```python
from build123d import *

# Parameters (mm, degrees)
F0_W      = 48.26
F0_H      = 35.56
F0_R      = 1.5
F1_DEPTH  = 2
F2_W      = 48.329203
F2_H      = 2
F3_DEPTH  = 25
F5_W      = 18
F5_H      = 9
F6_DEPTH  = 25
F7_W      = 40
F7_H      = 4
F8_DEPTH  = 25
F9_W      = 40
F9_H      = 20
F10_DEPTH = 3
F11_R     = 6.935469
F12_DEPTH = 30
F13_DEPTH = 25


with BuildPart() as f1:
    # F0 (on Top) → F1 (new body)
    with BuildSketch(Plane.XY):
        with Locations((0.875274, -1.180254)):
            Rectangle(F0_W, F0_H)
        with Locations((-13.254726, -14.960254)):
            Circle(F0_R, mode=Mode.SUBTRACT)
        with Locations((15.005274, -14.960254)):
            Circle(F0_R, mode=Mode.SUBTRACT)
        with Locations((-13.254726, 12.599746)):
            Circle(F0_R, mode=Mode.SUBTRACT)
        with Locations((15.005274, 12.599746)):
            Circle(F0_R, mode=Mode.SUBTRACT)
    extrude(amount=F1_DEPTH)

    # F2 (on Top) → F3 (join)
    with BuildSketch(Plane.XY):
        with Locations((0.840673, -19.942636)):
            Rectangle(F2_W, F2_H)
    extrude(amount=F3_DEPTH)

    # F5 (on face) → F6 (cut)
    with BuildSketch(Plane(origin=(0, 0, 0), x_dir=(1, 0, 0), z_dir=(0, 0, -1))):
        with Locations((0.875274, 14.442636)):
            Rectangle(F5_W, F5_H)
    extrude(amount=-F6_DEPTH, mode=Mode.SUBTRACT)

    # F7 (on face) → F8 (join)
    with BuildSketch(Plane.XZ.offset(20.942636)):
        with Locations((0.840672, 14)):
            Rectangle(F7_W, F7_H)
    extrude(amount=F8_DEPTH)

    # F9 (on face) → F10 (join)
    with BuildSketch(Plane.XZ.offset(45.942636)):
        with Locations((0.840672, 14)):
            Rectangle(F9_W, F9_H)
    extrude(amount=F10_DEPTH)

    # F11 (on face) → F12 (cut)
    with BuildSketch(Plane.XZ.offset(20.942636)):
        with Locations((0.840672, 14)):
            Circle(F11_R)
    extrude(amount=F12_DEPTH, mode=Mode.SUBTRACT)

    # F11 (on face) → F13 (cut)
    with BuildSketch(Plane.XZ.offset(20.942636)):
        with Locations((0.840672, 14)):
            Circle(F11_R)
    extrude(amount=-F13_DEPTH, mode=Mode.SUBTRACT)


solid = f1.part
```
Work out the finished part from the listing and answer in its coordinate system (mm). A direction names the side the tool comes from. Coordinates: 2 decimals unless noted, no trailing zeros. Write each loop counter-clockwise with the first axis right and the second up, starting at its lowest first coordinate (ties: lowest second). Pieces come first, ordered by that corner, then holes. Notation, with made-up numbers: (-31.5, -19) - (21.5, -19) arc R14 cw to (21.5, -13) - close; hole circle Ø4 at (-34, -5). An arc over 180 degrees is marked (long way). Answer as a JSON object with one key per item and string values.
Q1. Given pin 1 Ø5 at (x, z) = (15.5, 9) entering from +Y; pin 2 Ø1 at (x, z) = (2.5, 1) entering from -Y; pin 3 Ø1.5 at (x, y) = (-10, -35) entering from +Z; pin 4 Ø2 at (y, z) = (9.5, 4.5) entering from +X, each flat-ended and moving along its own axis, determine where each tip first touches the part or whether it passes through.
Results list:
{"pin 1": "stops at y = -18.94", "pin 2": "stops at y = -20.94", "pin 3": "stops at z = 16", "pin 4": "passes through"}
Q2. Find section A-A (z = 4.75). Write down the section's boundary in (x, y).
Results list:
{"outline": "(-23.32, -20.94) - (25.01, -20.94) - (25.01, -18.94) - (-23.32, -18.94) - close; (-19.16, -48.94) - (20.84, -48.94) - (20.84, -45.94) - (-19.16, -45.94) - close"}
Q3. Find section B-B (y = -40.5). Write down the section's boundary in (x, z), plus the area to 3 significant figures.
Results list:
{"outline": "(-19.16, 12) - (-5.8, 12) arc R6.94 cw to (-5.8, 16) - (-19.16, 16) - close; (7.48, 12) - (20.84, 12) - (20.84, 16) - (7.48, 16) arc R6.94 cw to start", "area": "105 mm^2"}
Q4. Consider L1, parallel to Y at x = -13.5, z = 11.5; L2, parallel to X at y = -20.4, z = 14; L3, parallel to X at y = -33.75, z = 14. Determine where each line is inside the solid, lowest interval first. Write a range as from..to.
Results list:
{"L1": "y = -48.94..-45.94, -20.94..-18.94", "L2": "x = -23.32..-6.09, 7.78..25.01", "L3": "x = -19.16..-6.09, 7.78..20.84"}
Q5. For a pull along Y with two mould halves and no side action, classify faces 1 (the flat face through (-4, -48.943, 21)), 2 (the flat face through (-23.324, -20, 12)), 3 (the flat face through (-13, -33, 16)) as pulls with the +Y half, pulls with the -Y half, needs draft (parallel to the pull), parting line crosses it, or undercut.
Results list:
{"face 1": "pulls with the -Y half", "face 2": "needs draft", "face 3": "undercut"}
Q6. Find section C-C (z = 17.25). Write down the section's boundary in (x, y).
Results list:
{"outline": "(-23.32, -20.94) - (-5.29, -20.94) - (-5.29, -18.94) - (-23.32, -18.94) - close; (-19.16, -48.94) - (-5.29, -48.94) - (-5.29, -45.94) - (-19.16, -45.94) - close; (6.97, -48.94) - (20.84, -48.94) - (20.84, -45.94) - (6.97, -45.94) - close; (6.97, -20.94) - (25.01, -20.94) - (25.01, -18.94) - (6.97, -18.94) - close"}
Q7. Which of the six approach directions +Z, -Z, +X, -X, +Y, -Y give full straight-line access (tool end or side, diameter ignored) to faces 4 (the flat face through (1, -1, 2)), 5 (the flat face through (1, -47, 24)), 6 (the flat face through (1, -45.943, 6)), 7 (the flat face through (-23.255, -1, 1))?
Results list:
{"face 4": "+Z, +X, -X, +Y", "face 5": "+Z, +X, -X, -Y", "face 6": "-Z, +X, -X", "face 7": "+Z, -Z, -X, +Y"}
Q8. Find section D-D (x = 19). Write down the section's boundary in (y, z).
Results list:
{"outline": "(-48.94, 4) - (-45.94, 4) - (-45.94, 12) - (-20.94, 12) - (-20.94, 0) - (16.6, 0) - (16.6, 2) - (-18.94, 2) - (-18.94, 25) - (-20.94, 25) - (-20.94, 16) - (-45.94, 16) - (-45.94, 24) - (-48.94, 24) - close"}
